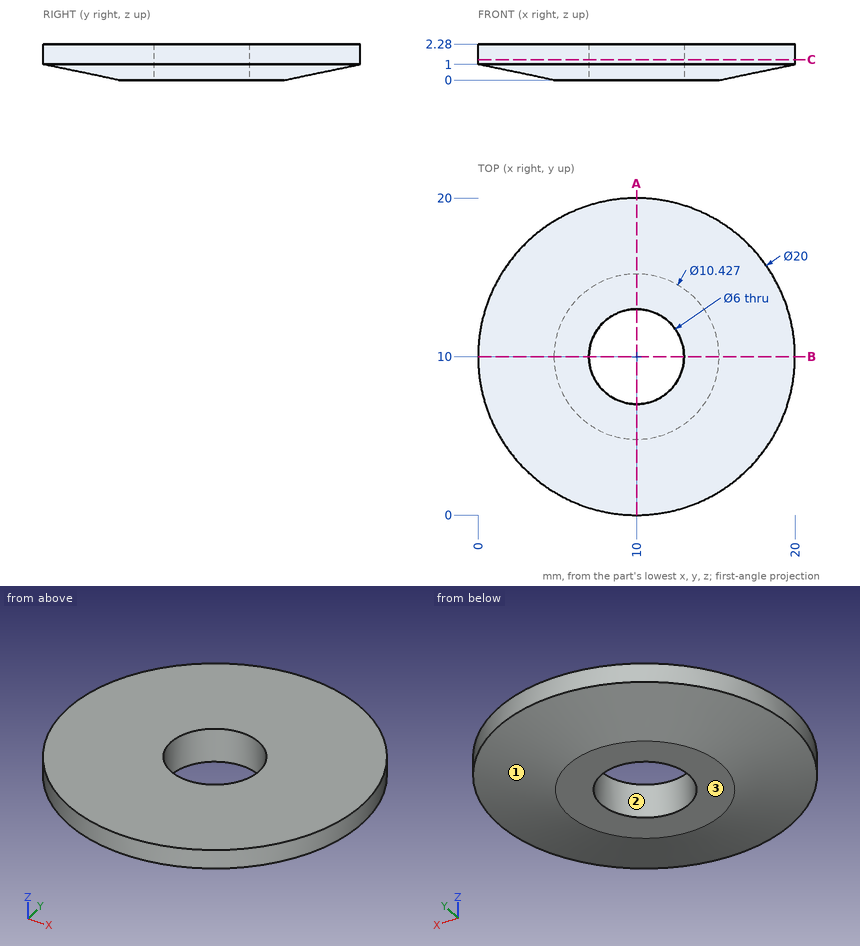
Job drawing, mm, ordinate dimensions from the low corner. One solid piece. Give positions to 0.01 mm unless a question says otherwise; leave off trailing zeros. Order: outer loops, then holes, each group sorted by start corner. A loop starts at its lowest first (then second) coordinate and runs counter-clockwise, first axis right, second up. Notation, with made-up numbers: M 41,86.5 L 85,86.5 A21 ccw 85,104.5 Z; hole C 75.25,2 d8. An arc over 180 degrees is marked long. Return JSON: item names as keys, results as strings.
Q1. Wall check: probe 1 along X at (y, z) = (10, 1.85); probe 2 along Y at (x, z) = (8.5, 2); probe 3 along X at (y, z) = (15.75, 1.25). Give the ranges that are in metal, low to high. Write a range as from..to.
Answer list:
{"probe 1": "x = 0..7, 13..20", "probe 2": "y = 0.11..7.4, 12.6..19.89", "probe 3": "x = 1.82..18.18"}
Q2. Band-saw the part on A-A (x = 10). Give the cut face in (y, z).
Answer list:
{"outline": "M 0,1 L 4.79,0 L 7,0 L 7,2.28 L 0,2.28 Z; M 13,0 L 15.21,0 L 20,1 L 20,2.28 L 13,2.28 Z"}
Q3. Two-plate mould, pull along Y, no slides. Class the marked faces 1, 2 and 3: pulls with the +Y half, pulls with the -Y half, needs draft (parallel to the pull), parting line crosses it, or undercut.
Answer list:
{"face 1": "parting line crosses it", "face 2": "undercut", "face 3": "needs draft"}
Q4. Flat gauge pins, fed straight in: pin 1 (1 mm diameter, centred on y = 14.5, z = 1, fed in from +X) (1 decimal); pin 2 (1 mm diameter, centred on x = 3, z = 1, fed in from -Y). Where does each tip first touch, or does it go through?
Answer list:
{"pin 1": "stops at x = 19.2", "pin 2": "stops at y = 2.4"}
Q5. Band-saw the part on C-C (z = 1.3). Give the cut face in (x, y).
Answer list:
{"outline": "C 10,10 d20; hole C 10,10 d6"}
